Autodesk Inventor part; units mm, degrees
ref_plane "YZ Plane" through (0, 0, 0) normal (1, 0, 0) x (0, 1, 0)
ref_plane "XZ Plane" through (0, 0, 0) normal (0, 1, 0) x (-1, 0, 0)
ref_plane "XY Plane" through (0, 0, 0) normal (0, 0, 1) x (1, 0, 0)
sketch "Sketch1" plane through (0, 0, 0) normal (0, 1, 0) x (-1, 0, 0)
  line L0 (14.5, 12.75) -> (-14.5, 12.75)
  line L1 (-14.5, 12.75) -> (-14.5, -12.75)
  line L2 (-14.5, -12.75) -> (14.5, -12.75)
  line L3 (14.5, -12.75) -> (14.5, 12.75)
  line L4 (14.5, 12.75) -> (-14.5, -12.75) construction
  line L5 (-14.5, 12.75) -> (14.5, -12.75) construction
  point P0 (0, 0)
  dimension "d0" = 29
  dimension "d1" = 25.5
extrude "Extrusion1" add sketch "Sketch1" along normal mid plane 3
sketch "Sketch2" plane through (0, 1.5, 0) normal (0, 1, 0) x (1, 0, 0)
  circle A0 centre (-10.75, 10) radius 1.5
  line L0 (14.5, 12.75) -> (-14.5, 12.75)
  line L1 (-14.5, 12.75) -> (-14.5, -12.75)
  circle A1 centre (10.75, 10) radius 1.5
  circle A2 centre (-10.75, -10) radius 1.5
  circle A3 centre (10.75, -10) radius 1.5
  point P0 (0, 0)
  dimension "d4" = 3
  dimension "d5" = 2.75
  dimension "d6" = 3.75
  dimension "d9" = 21.5
  dimension "d12" = 20
sketch "Sketch3" plane through (0, 1.5, 0) normal (0, 1, 0) x (1, 0, 0)
  circle A0 centre (0, 0) radius 7.25
  dimension "d15" = 14.5
extrude "Extrusion2" cut sketch "Sketch2" against normal through all
sketch "Sketch4" plane through (0, 1.5, 0) normal (0, 1, 0) x (1, 0, 0)
  line L0 (-5.4078, 7.0301) -> (8.8628, 7.0301) construction
  line L1 (8.8628, 7.0301) -> (8.8628, -8.322) construction
  line L2 (8.8628, -8.322) -> (-5.4078, -8.322) construction
  line L3 (-5.4078, -8.322) -> (-5.4078, 7.0301) construction
  spline S0 degree 2 poles (-0.467, -6.4334) (-1.8786, -6.4334) (-3.8592, -5.8434) (-4.7336, -5.4221) knots 0 0 0 1 2 2 2
  line L4 (-4.7336, -5.4221) -> (-4.7336, -3.2519)
  line L5 (-4.7336, -3.2519) -> (-4.6072, -3.2519)
  spline S1 degree 2 poles (-4.6072, -3.2519) (-3.7538, -4.0525) (-1.5942, -4.9374) (-0.5934, -4.9374) knots 0 0 0 1 2 2 2
  spline S2 degree 2 poles (-0.5934, -4.9374) (0.8394, -4.9374) (2.3037, -3.747) (2.3037, -2.7673) knots 0 0 0 1 2 2 2
  spline S3 degree 2 poles (2.3037, -2.7673) (2.3037, -1.9877) (1.5347, -1.0185) (0.7024, -0.7762) knots 0 0 0 1 2 2 2
  spline S4 degree 2 poles (0.7024, -0.7762) (0.1019, -0.6076) (-0.8989, -0.3759) (-1.6469, -0.1862) knots 0 0 0 1 2 2 2
  spline S5 degree 2 poles (-1.6469, -0.1862) (-2.3211, -0.0071) (-3.3851, 0.5301) (-3.796, 0.9621) knots 0 0 0 1 2 2 2
  spline S6 degree 2 poles (-3.796, 0.9621) (-4.1963, 1.394) (-4.6388, 2.5528) (-4.6388, 3.3113) knots 0 0 0 1 2 2 2
  spline S7 degree 2 poles (-4.6388, 3.3113) (-4.6388, 4.8916) (-2.1736, 7.0301) (-0.2668, 7.0301) knots 0 0 0 1 2 2 2
  spline S8 degree 2 poles (-0.2668, 7.0301) (0.8288, 7.0301) (2.7672, 6.5982) (3.5995, 6.1873) knots 0 0 0 1 2 2 2
  line L6 (3.5995, 6.1873) -> (3.5995, 4.1225)
  line L7 (3.5995, 4.1225) -> (3.4731, 4.1225)
  spline S9 degree 2 poles (3.4731, 4.1225) (2.8515, 4.6914) (0.9131, 5.5342) (-0.1509, 5.5342) knots 0 0 0 1 2 2 2
  spline S10 degree 2 poles (-0.1509, 5.5342) (-1.3519, 5.5342) (-2.8373, 4.407) (-2.8373, 3.4904) knots 0 0 0 1 2 2 2
  spline S11 degree 2 poles (-2.8373, 3.4904) (-2.8373, 2.6687) (-1.9629, 1.689) (-1.1412, 1.4677) knots 0 0 0 1 2 2 2
  spline S12 degree 2 poles (-1.1412, 1.4677) (-0.5934, 1.3203) (0.9974, 0.941) (1.5241, 0.783) knots 0 0 0 1 2 2 2
  spline S13 degree 2 poles (1.5241, 0.783) (2.8621, 0.3721) (4.1052, -1.2819) (4.1052, -2.4934) knots 0 0 0 1 2 2 2
  spline S14 degree 2 poles (4.1052, -2.4934) (4.1052, -3.2624) (3.4836, -4.7373) (2.9253, -5.2535) knots 0 0 0 1 2 2 2
  spline S15 degree 2 poles (2.9253, -5.2535) (2.3037, -5.8224) (0.7235, -6.4334) (-0.467, -6.4334) knots 0 0 0 1 2 2 2
  point P0 (0, 0)
extrude "Extrusion3" cut sketch "Sketch3" against normal blind 0.5
extrude "Extrusion4" add sketch "Sketch4" against normal blind 0.5
properties material "Iron, Cast"
Design review of the part built by this model. Coordinates are the model's own, in mm. A direction names the side the tool comes from. Coordinates: 2 decimals unless noted, no trailing zeros. Order: outer loops, then holes, each group sorted by start corner. A loop starts at its lowest first (then second) coordinate and runs counter-clockwise, first axis right, second up. Notation, with made-up numbers: (89, -28.5) - (134, -28.5) arc R14 cw to (134, -11.5) - close; hole circle Ø1 at (74.5, 82). An arc over 180 degrees is marked (long way). One line per question, with ' | ' between items.
Q1. Consider section C-C, the plane y = -0.15. Give the boundary of the cut face in (x, z).
Answer key:
outline: (-14.5, -12.75) - (14.5, -12.75) - (14.5, 12.75) - (-14.5, 12.75) - close; hole circle Ø3 at (-10.75, -10); hole circle Ø3 at (-10.75, 10); hole circle Ø3 at (10.75, -10); hole circle Ø3 at (10.75, 10)
Q2. Consider section B-B, the plane x = 10.75. Give the boundary of the cut face in (y, z).
Answer key:
outline: (-1.5, -12.75) - (1.5, -12.75) - (1.5, -11.5) - (-1.5, -11.5) - close; (-1.5, -8.5) - (1.5, -8.5) - (1.5, 8.5) - (-1.5, 8.5) - close; (-1.5, 11.5) - (1.5, 11.5) - (1.5, 12.75) - (-1.5, 12.75) - close
Q3. Clearance check with a flat-ended pin moving along its axis: pin 1 Ø5 at (x, z) = (-10.75, -10) entering from -Y. State where the tip first meets the part, or that it passes through.
Answer key:
pin 1: stops at y = -1.5
Q4. Consider section A-A, the plane z = -10. Give the boundary of the cut face in (x, y).
Answer key:
outline: (-14.5, -1.5) - (-12.25, -1.5) - (-12.25, 1.5) - (-14.5, 1.5) - close; (-9.25, -1.5) - (9.25, -1.5) - (9.25, 1.5) - (-9.25, 1.5) - close; (12.25, -1.5) - (14.5, -1.5) - (14.5, 1.5) - (12.25, 1.5) - close
Q5. The part is to be moulded in two halves that separate along X. For faces 3 (the flat face through (0, -1.5, 0)), 4 (the flat face through (14.5, 0, 0)), 5 (the cylindrical face through (9.56, 0.02, 10.91)), say which applies: +X half, -X half, draft (parallel to the pull), parting line (faces both ways), or undercut.
Answer key:
face 3: draft | face 4: +X half | face 5: undercut
Q6. For faces 1 (the flat face through (0, 0, -12.75)), 2 (the cylindrical face through (3.35, 1.25, 6.43)), list the 3-axis set-ups (+Z, -Z, +X, -X, +Y, -Y) from which the entire face can be reached by the end or side of a thin tool; tool diameter is ignored.
Answer key:
face 1: -Z, +X, -X, +Y, -Y | face 2: +Y
Q7. To check wall thickness, follow line 1 along X through (y, z) = (0.5, -10); line 2 along Z through (x, y) = (-10.75, 0.75); line 3 along X through (y, z) = (-1.35, 9.25). State the ranges of each line that lie inside material, in increasing order.
Answer key:
line 1: x = -14.5 to -12.25, -9.25 to 9.25, 12.25 to 14.5 | line 2: z = -12.75 to -11.5, -8.5 to 8.5, 11.5 to 12.75 | line 3: x = -14.5 to -12.05, -9.45 to 9.45, 12.05 to 14.5
